Can you work these out from the model? Positions are in its coordinate system, mm. Face numbers are marked on the shaded views. Round coordinates to 2 decimals unless told otherwise and drop trailing zeros. Loops run counter-clockwise (first coordinate to the right, second up) from the corner with the lowest first, then second, coordinate; pieces in that order, holes last.
(1) I want a section at B-B on z = 0.5. Write out the boundary of the cut face in (x, y) (3 decimals), plus the area to 3 significant figures.
(2) Thinking about a two-plate mould opening in X: for the marked faces 1, 2, 3 and 4, which applies, released by +X, released by -X, zero draft, split by the parting line, or undercut?
(3) Will this pin go through, and if not, where does the flat tip stop? pin 1 Ø2 at (x, y) = (-6.74, -166.65) entering from +Z.
(4) I want a section at C-C on x = 12.7. Write out the boundary of the cut face in (y, z), plus the area to 3 significant figures.
(5) If I drill on line 1 along Y through (x, z) = (0, 1); line 2 along Y through (x, z) = (-12.7, 1.75); line 3 along X through (y, z) = (-168.75, 1.15) (3 decimals), over which ranges is the centre line in solid material (lowest first)?
(6) I want a section at D-D on y = -160.5. Write out the boundary of the cut face in (x, z).
(7) I want a section at A-A on x = 0. Write out the boundary of the cut face in (y, z).
from build123d import *

# Parameters (mm, degrees)
SKETCH1_W             = 31.75
SKETCH1_H             = 12.7
BOSS_EXTRUDE1_DEPTH   = 2.286
FILLET1_R             = 2.54
SKETCH2_R             = 3.175
SKETCH2_R_2           = 1.1049
CUT_EXTRUDE1_DEPTH    = 3.286
F_2_CLEARANCE_HOLE1_D = 2.7051


with BuildPart() as part:
    # Sketch1 → Boss-Extrude1 (new body)
    with BuildSketch(Plane.XY):
        with Locations((-1.87e-07, -166.116000205)):
            Rectangle(SKETCH1_W, SKETCH1_H)
    extrude(amount=BOSS_EXTRUDE1_DEPTH)

    # Fillet1
    fillet1_edges = [part.edges().sort_by_distance(p)[0] for p in [
        (15.874999813, -172.466000205, 1.143),
        (-15.875000187, -172.466000205, 1.143),
        (-15.875000187, -159.766000205, 1.143),
        (15.874999813, -159.766000205, 1.143),
    ]]
    fillet(fillet1_edges, radius=FILLET1_R)

    # Sketch2 → Cut-Extrude1 (cut, through all)
    with BuildSketch(Plane.XY.offset(2.286)):
        with Locations((-1.87e-07, -166.116000205)):
            Circle(SKETCH2_R)
        with Locations((-6.735572471, -166.64610111)):
            Circle(SKETCH2_R_2)
    extrude(amount=-CUT_EXTRUDE1_DEPTH, mode=Mode.SUBTRACT)

    # #2 Clearance Hole1 (through all)
    with Locations(Plane.XY.offset(2.286)):
        with Locations((12.699999906, -166.116000205), (-12.700000094, -166.116000205)):
            Hole(F_2_CLEARANCE_HOLE1_D / 2)


solid = part.part
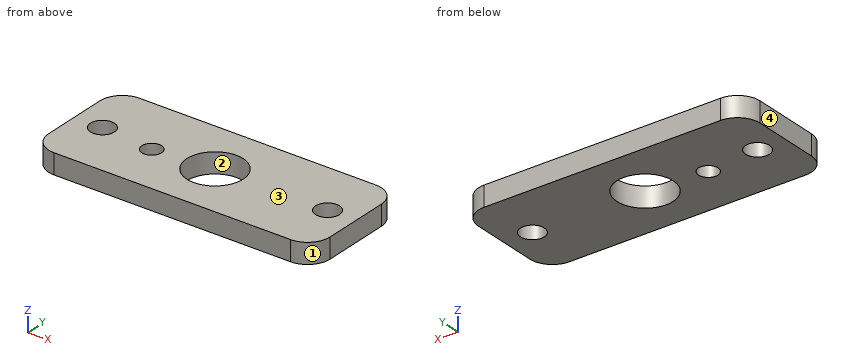
Filled sheet:
1. outline: (-15.875, -169.926) arc R2.54 ccw to (-13.335, -172.466) - (13.335, -172.466) arc R2.54 ccw to (15.875, -169.926) - (15.875, -162.306) arc R2.54 ccw to (13.335, -159.766) - (-13.335, -159.766) arc R2.54 ccw to (-15.875, -162.306) - close; hole circle Ø2.705 at (-12.7, -166.116); hole circle Ø2.21 at (-6.736, -166.646); hole circle Ø6.35 at (0, -166.116); hole circle Ø2.705 at (12.7, -166.116)
1. area: 351 mm2
2. face 1: released by +X
2. face 2: undercut
2. face 3: zero draft
2. face 4: released by -X
3. pin 1: passes through
4. outline: (-172.47, 0) - (-167.47, 0) - (-167.47, 2.29) - (-172.47, 2.29) - close; (-164.76, 0) - (-159.77, 0) - (-159.77, 2.29) - (-164.76, 2.29) - close
4. area: 22.8 mm2
5. line 1: y = -172.47 to -169.29, -162.94 to -159.77
5. line 2: y = -172.47 to -167.47, -164.76 to -159.77
5. line 3: x = -15.875 to -1.773, 1.773 to 15.875
6. outline: (-15.12, 0) - (15.12, 0) - (15.12, 2.29) - (-15.12, 2.29) - close
7. outline: (-172.47, 0) - (-169.29, 0) - (-169.29, 2.29) - (-172.47, 2.29) - close; (-162.94, 0) - (-159.77, 0) - (-159.77, 2.29) - (-162.94, 2.29) - close
